Work out the finished part from the listing and answer in its coordinate system (mm). Face numbers are marked on the shaded views. A direction names the side the tool comes from. Coordinates: 2 decimals unless noted, no trailing zeros. Write each loop counter-clockwise with the first axis right and the second up, starting at its lowest first coordinate (ties: lowest second). Pieces come first, ordered by that corner, then holes. Notation, with made-up numbers: (-9, 74.5) - (13, 74.5) arc R15 ccw to (13, 96.5) - close; hole circle Ø5 at (34, -6.75). An arc over 180 degrees is marked (long way). Use a Markdown table: item, result. Add a question column.
(1) The part is cut by section C-C, the plane z = -41. Give the vertices of the cut face in (x, y).
(2) A tool of negligible diameter and unlimited length cuts with its end or side. For the marked faces 1, 2 and 3, from which of +Z, -Z, +X, -X, +Y, -Y can it reach the whole face along a straight path? Write none if from no direction.
(3) The part is cut by section A-A, the plane x = -42.5. Give the vertices of the cut face in (y, z).
(4) The part is cut by section D-D, the plane x = 6. State how many separate pieces and enclosed holes the cut face has, then the cut area to 3 significant figures.
(5) Find the intervals of material crossed by line 1 (Z direction, x = 47, y = 4.75); line 2 (Y direction, x = -53, z = 44.5); line 3 (Z direction, x = -25.5, y = -3), in increasing order. Write a range as from..to.
(6) The part is cut by section B-B, the plane y = 9.75. Give the vertices of the cut face in (x, z).
(7) Given pin 1 Ø2 at (x, y) = (74.5, 0) entering from -Z; pin 2 Ø8 at (y, z) = (-7, 2.5) entering from +X; pin 3 Ø1.5 at (x, y) = (-14, -0.5) entering from -Z; pin 4 Ø2.5 at (x, y) = (-1, 1.5) entering from -Z, each flat-ended and moving along its own axis, determine where each tip first touches the part or whether it passes through.
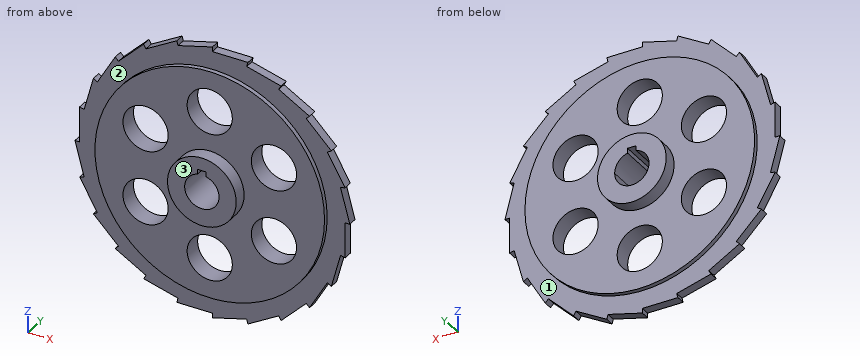
from build123d import *

# Parameters (mm, degrees)
F0_R     = 63.5
F1_DEPTH = 2.5
F2_R     = 63.5
F2_R_2   = 12.5
F2_R_3   = 19
F3_DEPTH = 5
F4_R     = 19
F5_DEPTH = 12.5


with BuildPart() as f1:
    # F0 (on Front) → F1 (new body, symmetric)
    with BuildSketch(Plane.XZ):
        Polygon((76, 0), (70.908965, 19), (73.410363, 19.670247), (63.575239, 36.705181), (65.817931, 38), (51.908965, 51.908965), (53.740115, 53.740115), (36.705181, 63.575239), (38, 65.817931), (19, 70.908965), (19.670247, 73.410363), (0, 73.410363), (0, 76), (-19, 70.908965), (-19.670247, 73.410363), (-36.705181, 63.575239), (-38, 65.817931), (-51.908965, 51.908965), (-53.740115, 53.740115), (-63.575239, 36.705181), (-65.817931, 38), (-70.908965, 19), (-73.410363, 19.670247), (-73.410363, 0), (-76, 0), (-70.908965, -19), (-73.410363, -19.670247), (-63.575239, -36.705181), (-65.817931, -38), (-51.908965, -51.908965), (-53.740115, -53.740115), (-36.705181, -63.575239), (-38, -65.817931), (-19, -70.908965), (-19.670247, -73.410363), (0, -73.410363), (0, -76), (19, -70.908965), (19.670247, -73.410363), (36.705181, -63.575239), (38, -65.817931), (51.908965, -51.908965), (53.740115, -53.740115), (63.575239, -36.705181), (65.817931, -38), (70.908965, -19), (73.410363, -19.670247), (73.410363, 0), align=None)
        Circle(F0_R, mode=Mode.SUBTRACT)
    extrude(amount=F1_DEPTH, both=True)

    # F2 (on Front) → F3 (join, symmetric)
    with BuildSketch(Plane.XZ):
        Circle(F2_R)
        with Locations((-35.507042, -20.5)):
            Circle(F2_R_2, mode=Mode.SUBTRACT)
        with Locations((0, -41)):
            Circle(F2_R_2, mode=Mode.SUBTRACT)
        with Locations((35.507042, -20.5)):
            Circle(F2_R_2, mode=Mode.SUBTRACT)
        with Locations((-35.507042, 20.5)):
            Circle(F2_R_2, mode=Mode.SUBTRACT)
        Circle(F2_R_3, mode=Mode.SUBTRACT)
        with Locations((35.507042, 20.5)):
            Circle(F2_R_2, mode=Mode.SUBTRACT)
        with Locations((0, 41)):
            Circle(F2_R_2, mode=Mode.SUBTRACT)
    extrude(amount=F3_DEPTH, both=True)

    # F4 (on Front) → F5 (join, symmetric)
    with BuildSketch(Plane.XZ):
        Circle(F4_R)
        with BuildLine():
            ThreePointArc((2.38, 9.197043), (7.51199, 5.815497), (9.5, 0))
            ThreePointArc((9.5, 0), (-5.815497, -7.51199), (-2.38, 9.197043))
            Line((-2.38, 9.197043), (-2.38, 11.88))
            Line((-2.38, 11.88), (0, 11.88))
            Line((0, 11.88), (2.38, 11.88))
            Line((2.38, 11.88), (2.38, 9.197043))
        make_face(mode=Mode.SUBTRACT)
    extrude(amount=F5_DEPTH, both=True)


solid = f1.part
Model answer:
| question | item | result |
|---|---|---|
| 1 | outline | (-62.82, -2.5) - (-48.49, -2.5) - (-48.49, -5) - (-12.5, -5) - (-12.5, 5) - (-48.49, 5) - (-48.49, 2.5) - (-62.82, 2.5) - close; (12.5, -5) - (48.49, -5) - (48.49, -2.5) - (61.1, -2.5) - (61.1, 2.5) - (48.49, 2.5) - (48.49, 5) - (12.5, 5) - close |
| 2 | face 1 | +Y |
| 2 | face 2 | -Y |
| 2 | face 3 | +Z, -Z, +X, -X, -Y |
| 3 | outline | (-5, -47.18) - (-2.5, -47.18) - (-2.5, -60.23) - (2.5, -60.23) - (2.5, -47.18) - (5, -47.18) - (5, -30.86) - (-5, -30.86) - close; (-5, -10.14) - (5, -10.14) - (5, 10.14) - (-5, 10.14) - close; (-5, 30.86) - (5, 30.86) - (5, 47.18) - (2.5, 47.18) - (2.5, 61.32) - (-2.5, 61.32) - (-2.5, 47.18) - (-5, 47.18) - close |
| 4 | separate pieces | 4 |
| 4 | enclosed holes | 0 |
| 4 | area | 1,110 mm^2 |
| 5 | line 1 | -42.7..-25.42, -15.58..15.58, 25.42..42.7 |
| 5 | line 2 | -2.5..2.5 |
| 5 | line 3 | -58.15..-27.99, -13.01..13.01, 27.99..58.15 |
| 6 | outline | circle Ø38 at (0, 0); hole (-2.38, 9.2) arc R9.5 ccw (long way) to (2.38, 9.2) - (2.38, 11.88) - (-2.38, 11.88) - close |
| 7 | pin 1 | z = 0 |
| 7 | pin 2 | x = 63.5 |
| 7 | pin 3 | z = -73.41 |
| 7 | pin 4 | z = -76 |
